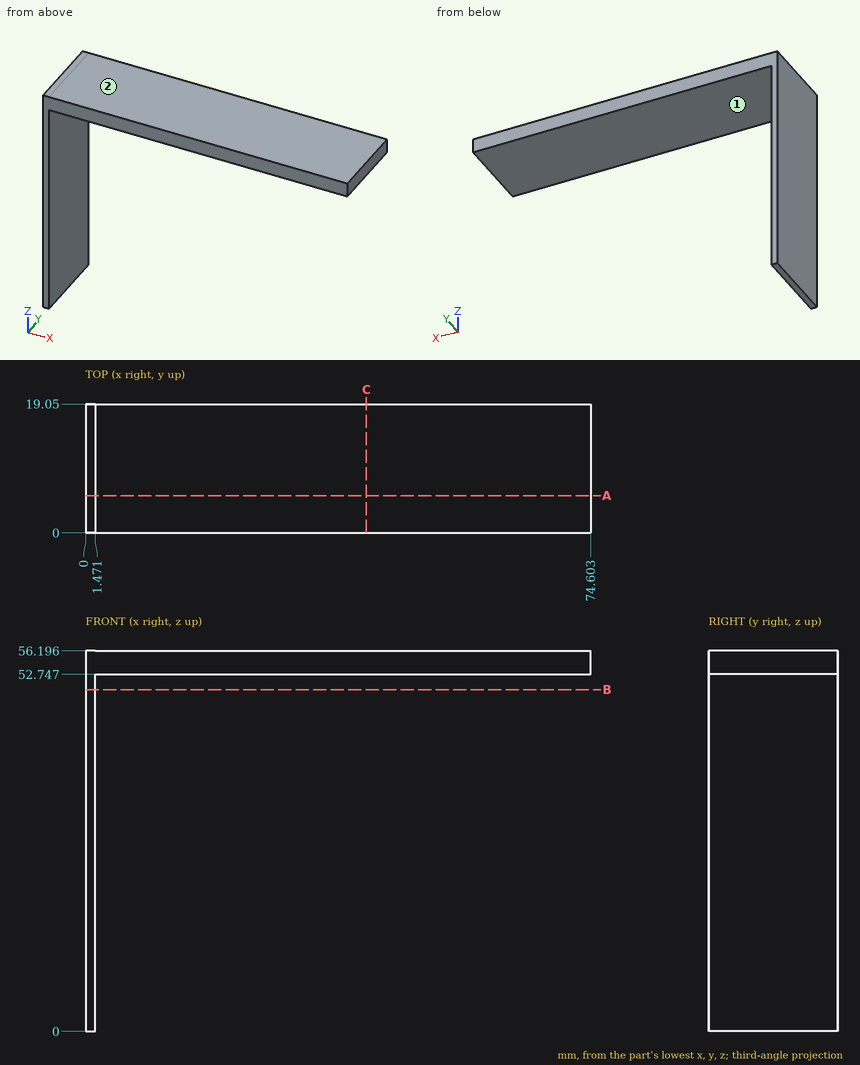
Source: three-view drawing plus pictorial views. Frame: mm from the lowest corner of the part. A direction names the side the tool comes from. Round coordinates to 2 decimals unless told otherwise and drop trailing zeros. Loops run counter-clockwise (first coordinate to the right, second up) from the corner with the lowest first, then second, coordinate; pieces in that order, holes last. Notation, with made-up numbers: (5.5, 5.25) - (35.5, 5.25) arc R10 cw to (35.5, 14.25) - close; hole circle Ø5 at (59, 23). An arc over 180 degrees is marked (long way). Write item = value, one per line. Start each with the question number.
Item 1: Section query B-B on z = 50.5. Output: boundary loops of the cut face in (x, y).
Item 2: First-contact query: pin 1 Ø8 at (x, y) = (26, 9.5) entering from -Z; pin 2 Ø9.5 at (y, z) = (6, 39) entering from +X. Flat tips, straight axial feed; report the tip coordinate or a pass-through.
Item 3: Material intervals for line 1 (Z direction, x = 25.5, y = 16.5); line 2 (X direction, y = 12.25, z = 11.5), sorted ascending.
Item 4: Reachability of the marked faces 1 and 2 from +Z, -Z, +X, -X, +Y, -Y: full face, straight path, thin tool, end or side. Return the list, or none.
Item 5: Section query C-C on x = 41.5. Output: boundary loops of the cut face in (y, z), plus the area to 3 significant figures.
Item 6: Section query A-A on y = 5.5. Output: boundary loops of the cut face in (x, z), plus the area to 3 significant figures.
Results list:
q1.outline = (0, 0) - (1.47, 0) - (1.47, 19.05) - (0, 19.05) - close
q2.pin_1 = 52.75
q2.pin_2 = 1.47
q3.line_1 = 52.75 to 56.2
q3.line_2 = 0 to 1.47
q4.face_1 = -Z, +X, +Y, -Y
q4.face_2 = +Z, +X, -X, +Y, -Y
q5.outline = (0, 52.75) - (19.05, 52.75) - (19.05, 56.2) - (0, 56.2) - close
q5.area = 65.7 mm²
q6.outline = (0, 0) - (1.47, 0) - (1.47, 52.75) - (74.6, 52.75) - (74.6, 56.2) - (0, 56.2) - close
q6.area = 335 mm²
